Design review of the part built by this model. Coordinates are the model's own, in mm. Face numbers are marked on the shaded views. A direction names the side the tool comes from. Round coordinates to 2 decimals unless told otherwise and drop trailing zeros. Order: outer loops, then holes, each group sorted by start corner. A loop starts at its lowest first (then second) coordinate and runs counter-clockwise, first axis right, second up. Notation, with made-up numbers: (16, -26) - (34, -26) arc R9 cw to (34, -22) - close; hole circle Ø3 at (-10.75, 59.25). An arc over 180 degrees is marked (long way). Answer as a JSON object with one key per item and string values. Group by question number.
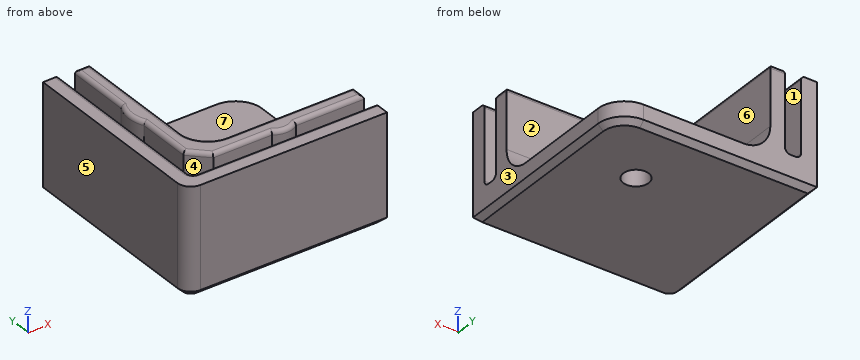
from build123d import *

# Parameters (mm, degrees)
F0_W          = 38.1
F0_H          = 38.1
F1_DEPTH      = 20.32
F2_W          = 29.21
F2_H          = 29.21
F3_DEPTH      = 16.51
F5_DEPTH      = 15.24
F6_T1_DEPTH   = 29.21
F7_R          = 5.08
F8_R          = 5.08
F9_R          = 2.54
F10_R         = 2.413
F11_DEPTH     = 20.321
F13_DEPTH     = 15.24
F14_T1_DEPTH  = 14.224
F14_T3_DEPTH  = 34.036
F14_T5_DEPTH  = 34.036
F14_T7_DEPTH  = 19.05
F14_T9_DEPTH  = 18.3199171099
F14_S13_W     = 1.03632
F14_S13_H     = 1.03632
F14_T14_DEPTH = 1.03632
F14_T20_DEPTH = 16.861733183
F14_T26_DEPTH = 22.6379171099
F14_T31_DEPTH = 23.368
F14_T36_ANGLE = 257.1357278548
F14_T42_DEPTH = 16.861733183
F14_T46_DEPTH = 23.368
F14_T53_DEPTH = 16.861733183
F14_T57_DEPTH = 22.6379171099
F15_SIZE      = 1.016
F16_R         = 0.762


# Not quite as in the source:
# - a fillet or chamfer that OpenCascade refuses, or shapes differently, is made with other operations: its cross-section is extruded or revolved along the edge and cut away or added


with BuildPart() as f1:
    # F0 (on Top) → F1 (new body)
    with BuildSketch(Plane.XY):
        with Locations((19.05, 19.05)):
            Rectangle(F0_W, F0_H)
    extrude(amount=F1_DEPTH)

    # F2 (on face) → F3 (cut)
    with BuildSketch(Plane.XY.offset(20.32)):
        with Locations((23.495, 23.495)):
            Rectangle(F2_W, F2_H)
    extrude(amount=-F3_DEPTH, mode=Mode.SUBTRACT)

    # F4 (on face) → F5 (cut)
    with BuildSketch(Plane.XY.offset(20.32)):
        Polygon((6.096, 38.1), (3.048, 38.1), (3.048, 3.048), (38.1, 3.048), (38.1, 6.096), (9.398, 6.096), (6.096, 6.096), (6.096, 9.398), align=None)
        Polygon((9.398, 6.096), (6.096, 9.398), (6.096, 6.096), align=None)
    extrude(amount=-F5_DEPTH, mode=Mode.SUBTRACT)

    # F6: fillet of radius 5.08 on 1 edges, made by hand

    # F6_s2 → F6_t1 (cut)
    with BuildSketch(Plane.XY.offset(-12.7)):
        with BuildLine():
            ThreePointArc((33.02, 38.1), (36.6121024484, 36.6121024484), (38.1, 33.02))
            Line((38.1, 33.02), (38.1, 38.1))
            Line((38.1, 38.1), (33.02, 38.1))
        make_face()
    extrude(amount=F6_T1_DEPTH, mode=Mode.SUBTRACT)

    # F7
    f7_edges = [f1.edges().sort_by_distance(p)[0] for p in [
        (8.89, 8.89, 12.065),
    ]]
    fillet(f7_edges, radius=F7_R)

    # F8
    f8_edges = [f1.edges().sort_by_distance(p)[0] for p in [
        (26.035, 8.89, 3.81),
        (10.377898, 10.377898, 3.81),
        (8.89, 26.035, 3.81),
    ]]
    fillet(f8_edges, radius=F8_R)

    # F9
    f9_edges = [f1.edges().sort_by_distance(p)[0] for p in [
        (0, 0, 10.16),
    ]]
    fillet(f9_edges, radius=F9_R)

    # F10 (on face) → F11 (cut, through all)
    with BuildSketch(Plane(origin=(0, 0, 0), x_dir=(1, 0, 0), z_dir=(0, 0, -1))):
        with Locations((25.144717139, -25.144717139)):
            Circle(F10_R)
    extrude(amount=-F11_DEPTH, mode=Mode.SUBTRACT)

    # F12 (on face) → F13 (join, through all)
    with BuildSketch(Plane.XY.offset(20.32)):
        with BuildLine():
            Line((25.146, 6.096), (20.574, 6.096))
            ThreePointArc((20.574, 6.096), (22.86, 5.334), (25.146, 6.096))
        make_face()
        with BuildLine():
            Line((6.096, 19.8439171099), (6.096, 25.8760828901))
            ThreePointArc((6.096, 25.8760828901), (5.334, 22.86), (6.096, 19.8439171099))
        make_face()
    extrude(amount=-F13_DEPTH)

    # F14: fillet of radius 1.016 on 9 edges, made by hand

    # F14_s2 → F14_t1 (join)
    with BuildSketch(Plane.XY.offset(6.096)):
        with BuildLine():
            ThreePointArc((4.064, 3.048), (3.3455795103, 3.3455795103), (3.048, 4.064))
            Line((3.048, 4.064), (3.02768, 4.064))
            Line((3.02768, 4.064), (3.02768, 3.02768))
            Line((3.02768, 3.02768), (4.064, 3.02768))
            Line((4.064, 3.02768), (4.064, 3.048))
        make_face()
    extrude(amount=F14_T1_DEPTH)

    # F14_s4 → F14_t3 (join)
    with BuildSketch(Plane.YZ.offset(4.064)):
        with BuildLine():
            ThreePointArc((4.064, 5.08), (3.3455795103, 5.3775795103), (3.048, 6.096))
            Line((3.048, 6.096), (3.02768, 6.096))
            Line((3.02768, 6.096), (3.02768, 5.05968))
            Line((3.02768, 5.05968), (4.064, 5.05968))
            Line((4.064, 5.05968), (4.064, 5.08))
        make_face()
    extrude(amount=F14_T3_DEPTH)

    # F14_s6 → F14_t5 (join)
    with BuildSketch(Plane.XZ.offset(-38.1)):
        with BuildLine():
            ThreePointArc((4.064, 5.08), (3.3455795103, 5.3775795103), (3.048, 6.096))
            Line((3.048, 6.096), (3.02768, 6.096))
            Line((3.02768, 6.096), (3.02768, 5.05968))
            Line((3.02768, 5.05968), (4.064, 5.05968))
            Line((4.064, 5.05968), (4.064, 5.08))
        make_face()
    extrude(amount=F14_T5_DEPTH)

    # F14_s8 → F14_t7 (join)
    with BuildSketch(Plane.YZ.offset(19.05)):
        with BuildLine():
            ThreePointArc((6.096, 6.096), (5.7984204897, 5.3775795103), (5.08, 5.08))
            Line((5.08, 5.08), (5.08, 5.05968))
            Line((5.08, 5.05968), (6.11632, 5.05968))
            Line((6.11632, 5.05968), (6.11632, 6.096))
            Line((6.11632, 6.096), (6.096, 6.096))
        make_face()
    extrude(amount=F14_T7_DEPTH)

    # F14_s10 → F14_t9 (join)
    with BuildSketch(Plane.XZ.offset(-38.1)):
        with BuildLine():
            ThreePointArc((5.08, 5.08), (5.7984204897, 5.3775795103), (6.096, 6.096))
            Line((6.096, 6.096), (6.11632, 6.096))
            Line((6.11632, 6.096), (6.11632, 5.05968))
            Line((6.11632, 5.05968), (5.08, 5.05968))
            Line((5.08, 5.05968), (5.08, 5.08))
        make_face()
    extrude(amount=F14_T9_DEPTH)


with BuildPart() as f14_tool12:
    # F14_s13 → F14_t14 (new body)
    with BuildSketch(Plane.YZ.offset(4.064)):
        with Locations((3.54584, 5.57784)):
            Rectangle(F14_S13_W, F14_S13_H)
    extrude(amount=-F14_T14_DEPTH)

    # F14_s15 → F14_t16 (revolve, cut)
    with BuildSketch(Plane(origin=(4.064, 4.064, 6.096), x_dir=(0, 0.7071067812, 0.7071067812), z_dir=(0, -0.7071067812, 0.7071067812))):
        with BuildLine():
            ThreePointArc((0, -1.016), (1.016, 0), (0, 1.016))
            Line((0, 1.016), (0, -1.016))
        make_face()
    revolve(axis=Axis((4.064, 4.064, 6.096), (-1, 0, 0)), mode=Mode.SUBTRACT)


with BuildPart() as f1_1:
    add(f1.part)

    # F14_t11: union F14_tool12
    add(f14_tool12.part)


with BuildPart() as f14_tool18:
    # F14_s19 → F14_t20 (new body)
    with BuildSketch(Plane(origin=(5.9615229381, -5.9615229381, 0), x_dir=(0, 0, 1), z_dir=(-0.7071067812, 0.7071067812, 0))):
        with BuildLine():
            ThreePointArc((5.08, 9.9399124677), (5.3775795103, 10.6583329574), (6.096, 10.9559124677))
            Line((6.096, 10.9559124677), (6.096, 10.9762324677))
            Line((6.096, 10.9762324677), (5.05968, 10.9762324677))
            Line((5.05968, 10.9762324677), (5.05968, 9.9399124677))
            Line((5.05968, 9.9399124677), (5.08, 9.9399124677))
        make_face()
    extrude(amount=F14_T20_DEPTH)

    split(bisect_by=Plane.YZ.offset(6.096), keep=Keep.TOP)

    split(bisect_by=Plane.XZ.offset(-6.096), keep=Keep.BOTTOM)


with BuildPart() as f1_2:
    add(f1_1.part)

    # F14_t17: union F14_tool18
    add(f14_tool18.part)


with BuildPart() as f14_tool24:
    # F14_s25 → F14_t26 (new body)
    with BuildSketch(Plane.XZ.offset(-3.302)):
        with BuildLine():
            ThreePointArc((5.08, 5.08), (5.7984204897, 5.3775795103), (6.096, 6.096))
            Line((6.096, 6.096), (6.11632, 6.096))
            Line((6.11632, 6.096), (6.11632, 5.05968))
            Line((6.11632, 5.05968), (5.08, 5.05968))
            Line((5.08, 5.05968), (5.08, 5.08))
        make_face()
    extrude(amount=-F14_T26_DEPTH)

    split(bisect_by=Plane(origin=(7.747, 7.747, 0), x_dir=(0, 0, 1), z_dir=(0.7071067812, 0.7071067812, 0)), keep=Keep.TOP)


with BuildPart() as f1_3:
    add(f1_2.part)

    # F14_t23: union F14_tool24
    add(f14_tool24.part)


with BuildPart() as f14_tool29:
    # F14_s30 → F14_t31 (new body)
    with BuildSketch(Plane.YZ.offset(26.67)):
        with BuildLine():
            ThreePointArc((5.08, 5.08), (5.7984204897, 5.3775795103), (6.096, 6.096))
            Line((6.096, 6.096), (6.11632, 6.096))
            Line((6.11632, 6.096), (6.11632, 5.05968))
            Line((6.11632, 5.05968), (5.08, 5.05968))
            Line((5.08, 5.05968), (5.08, 5.08))
        make_face()
    extrude(amount=-F14_T31_DEPTH)

    split(bisect_by=Plane(origin=(7.747, 7.747, 0), x_dir=(0, 0, 1), z_dir=(0.7071067812, 0.7071067812, 0)), keep=Keep.TOP)


with BuildPart() as f1_4:
    add(f1_3.part)

    # F14_t28: union F14_tool29
    add(f14_tool29.part)


with BuildPart() as f14_tool34:
    # F14_s35 → F14_t36 (revolve)
    with BuildSketch(Plane(origin=(13.3424429627, 16.7330298048, 0), x_dir=(0, 0, 1), z_dir=(0.6234411592, 0.7818702712, 0))):
        with BuildLine():
            ThreePointArc((5.08, 7.3468084408), (5.3775795103, 8.0652289305), (6.096, 8.3628084408))
            Line((6.096, 8.3628084408), (6.096, 8.3831284408))
            Line((6.096, 8.3831284408), (5.05968, 8.3831284408))
            Line((5.05968, 8.3831284408), (5.05968, 7.3468084408))
            Line((5.05968, 7.3468084408), (5.08, 7.3468084408))
        make_face()
    revolve(axis=Axis((22.86, 9.144, 5.08), (0, 0, 1)), revolution_arc=F14_T36_ANGLE)

    split(bisect_by=Plane.XZ.offset(-6.096), keep=Keep.TOP)


with BuildPart() as f1_5:
    add(f1_4.part)

    # F14_t33: union F14_tool34
    add(f14_tool34.part)


with BuildPart() as f14_tool40:
    # F14_s41 → F14_t42 (new body)
    with BuildSketch(Plane(origin=(5.9615229381, -5.9615229381, 0), x_dir=(0, 0, 1), z_dir=(-0.7071067812, 0.7071067812, 0))):
        with BuildLine():
            ThreePointArc((5.08, 9.9399124677), (5.3775795103, 10.6583329574), (6.096, 10.9559124677))
            Line((6.096, 10.9559124677), (6.096, 10.9762324677))
            Line((6.096, 10.9762324677), (5.05968, 10.9762324677))
            Line((5.05968, 10.9762324677), (5.05968, 9.9399124677))
            Line((5.05968, 9.9399124677), (5.08, 9.9399124677))
        make_face()
    extrude(amount=F14_T42_DEPTH)

    split(bisect_by=Plane.XZ.offset(-6.096), keep=Keep.TOP)


with BuildPart() as f14_tool44:
    # F14_s45 → F14_t46 (new body)
    with BuildSketch(Plane.YZ.offset(26.67)):
        with BuildLine():
            ThreePointArc((5.08, 5.08), (5.7984204897, 5.3775795103), (6.096, 6.096))
            Line((6.096, 6.096), (6.11632, 6.096))
            Line((6.11632, 6.096), (6.11632, 5.05968))
            Line((6.11632, 5.05968), (5.08, 5.05968))
            Line((5.08, 5.05968), (5.08, 5.08))
        make_face()
    extrude(amount=-F14_T46_DEPTH)

    split(bisect_by=Plane(origin=(7.747, 7.747, 0), x_dir=(0, 0, 1), z_dir=(-0.7071067812, -0.7071067812, 0)), keep=Keep.TOP)


with BuildPart() as f14_tool40_1:
    add(f14_tool40.part)

    # F14_t48: intersect F14_tool44
    add(f14_tool44.part, mode=Mode.INTERSECT)


with BuildPart() as f1_6:
    add(f1_5.part)

    # F14_t38: union F14_tool40
    add(f14_tool40_1.part)


with BuildPart() as f14_tool51:
    # F14_s52 → F14_t53 (new body)
    with BuildSketch(Plane(origin=(5.9615229381, -5.9615229381, 0), x_dir=(0, 0, 1), z_dir=(-0.7071067812, 0.7071067812, 0))):
        with BuildLine():
            ThreePointArc((5.08, 9.9399124677), (5.3775795103, 10.6583329574), (6.096, 10.9559124677))
            Line((6.096, 10.9559124677), (6.096, 10.9762324677))
            Line((6.096, 10.9762324677), (5.05968, 10.9762324677))
            Line((5.05968, 10.9762324677), (5.05968, 9.9399124677))
            Line((5.05968, 9.9399124677), (5.08, 9.9399124677))
        make_face()
    extrude(amount=F14_T53_DEPTH)

    split(bisect_by=Plane.YZ.offset(6.096), keep=Keep.BOTTOM)


with BuildPart() as f14_tool55:
    # F14_s56 → F14_t57 (new body)
    with BuildSketch(Plane.XZ.offset(-3.302)):
        with BuildLine():
            ThreePointArc((5.08, 5.08), (5.7984204897, 5.3775795103), (6.096, 6.096))
            Line((6.096, 6.096), (6.11632, 6.096))
            Line((6.11632, 6.096), (6.11632, 5.05968))
            Line((6.11632, 5.05968), (5.08, 5.05968))
            Line((5.08, 5.05968), (5.08, 5.08))
        make_face()
    extrude(amount=-F14_T57_DEPTH)

    split(bisect_by=Plane(origin=(7.747, 7.747, 0), x_dir=(0, 0, 1), z_dir=(-0.7071067812, -0.7071067812, 0)), keep=Keep.TOP)


with BuildPart() as f14_tool51_1:
    add(f14_tool51.part)

    # F14_t59: intersect F14_tool55
    add(f14_tool55.part, mode=Mode.INTERSECT)


with BuildPart() as f1_7:
    add(f1_6.part)

    # F14_t49: union F14_tool51
    add(f14_tool51_1.part)

    # F15
    f15_edges = [f1_7.edges().sort_by_distance(p)[0] for p in [
        (20.32, 0, 0),
        (16.51, 38.1, 0),
        (36.612102, 36.612102, 0),
        (0.743949, 0.743949, 0),
        (38.1, 16.51, 0),
        (0, 20.32, 0),
    ]]
    chamfer(f15_edges, length=F15_SIZE)

    # F16
    f16_edges = [f1_7.edges().sort_by_distance(p)[0] for p in [
        (3.048, 21.082, 20.32),
        (31.623, 6.096, 20.32),
        (22.86, 5.334, 20.32),
        (8.89, 26.035, 20.32),
        (7.493, 38.1, 20.32),
        (6.096, 31.988041, 20.32),
        (5.334, 22.86, 20.32),
        (6.096, 14.620959, 20.32),
        (7.747, 7.747, 20.32),
        (14.986, 6.096, 20.32),
        (38.1, 7.493, 20.32),
        (26.035, 8.89, 20.32),
        (10.377898, 10.377898, 20.32),
        (21.082, 3.048, 20.32),
        (3.34558, 3.34558, 20.32),
    ]]
    fillet(f16_edges, radius=F16_R)


solid = f1_7.part
1. Mouldability with a two-part tool opening along X and no side actions: class the marked faces 4, 5, 6 and 7 as pulls with the +X half, pulls with the -X half, needs draft (parallel to the pull), parting line crosses it, or undercut.
2. Tool access review of the marked faces 1, 2 and 3: name each direction out of +Z, -Z, +X, -X, +Y, -Y from which nothing blocks a thin tool from reaching the whole face with its end or side.
3. Take a section at D-D, the plane z = 7.75. Give the boundary of the cut face in (x, y).
4. To check wall thickness, follow line 1 (X direction, y = 17, z = 11.5); line 2 (Y direction, x = 23, z = 15). State the ranges of each line that lie inside material, in increasing order. Write a range as from..to.
5. Clearance check with flat-ended pins moving along their axes: P1, Ø17, axis at x = 24.5, y = 28, coming from the +Z side; P2, Ø8, axis at x = 27.5, y = 13.5, coming from the +Z side; P3, Ø8.5, axis at x = 20, z = 15, coming from the +Y side. State where each tip first meets the part, or that it passes through.
6. Take a section at B-B, the plane y = 29.5. Give the boundary of the cut face in (x, z).
7. Take a section at A-A, the plane z = 10. Give the boundary of the cut face in (x, y), then the cut area to 3 significant figures.
Response values:
{
 "1": {"face 4": "undercut", "face 5": "pulls with the -X half", "face 6": "pulls with the +X half", "face 7": "needs draft"},
 "2": {"face 1": "+Z, +Y", "face 2": "+Z, +X, +Y", "face 3": "+Z, -Z, +X, +Y, -Y"},
 "3": {"outline": "(0, 2.54) arc R2.54 ccw to (2.54, 0) - (38.1, 0) - (38.1, 3.05) - (4.06, 3.05) arc R1.02 cw to (3.05, 4.06) - (3.05, 38.1) - (0, 38.1) - close; (6.1, 9.4) - (9.4, 6.1) - (20.57, 6.1) arc R3.81 ccw to (25.15, 6.1) - (38.1, 6.1) - (38.1, 9.02) - (13.97, 9.02) arc R4.95 cw to (9.02, 13.97) - (9.02, 38.1) - (6.1, 38.1) - (6.1, 25.88) arc R6.35 ccw to (6.1, 19.84) - close"},
 "4": {"line 1": "0..3.05, 6.1..8.89", "line 2": "0..3.05, 5.34..8.89"},
 "5": {"P1": "z = 3.81", "P2": "z = 6.48", "P3": "y = 8.89"},
 "6": {"outline": "(0, 1.02) - (1.02, 0) - (37.08, 0) - (38.1, 1.02) - (38.1, 3.81) - (13.97, 3.81) arc R5.08 cw to (8.89, 8.89) - (8.89, 19.56) arc R0.76 ccw to (8.13, 20.32) - (6.86, 20.32) arc R0.76 ccw to (6.1, 19.56) - (6.1, 6.1) arc R1.02 cw to (5.08, 5.08) - (4.06, 5.08) arc R1.02 cw to (3.05, 6.1) - (3.05, 19.56) arc R0.76 ccw to (2.29, 20.32) - (0, 20.32) - close"},
 "7": {"outline": "(0, 2.54) arc R2.54 ccw to (2.54, 0) - (38.1, 0) - (38.1, 3.05) - (4.06, 3.05) arc R1.02 cw to (3.05, 4.06) - (3.05, 38.1) - (0, 38.1) - close; (6.1, 9.4) - (9.4, 6.1) - (20.57, 6.1) arc R3.81 ccw to (25.15, 6.1) - (38.1, 6.1) - (38.1, 8.89) - (13.97, 8.89) arc R5.08 cw to (8.89, 13.97) - (8.89, 38.1) - (6.1, 38.1) - (6.1, 25.88) arc R6.35 ccw to (6.1, 19.84) - close", "area": "398 mm2"}
}
